Here's how the part is built. I have some questions about the finished solid (model axes, mm). Face numbers are marked on the shaded views. A direction names the side the tool comes from. Give positions to 0.01 mm unless a question says otherwise; leave off trailing zeros. Loops run counter-clockwise (first coordinate to the right, second up) from the corner with the lowest first, then second, coordinate; pieces in that order, holes last.
Q1. Will these pins go through, and if not, where does the flat tip stop? P1, Ø5, axis at y = 4, z = -1, coming from the +X side; P2, Ø1.2, axis at x = 30, y = 22, coming from the +Z side; P3, Ø6.5, axis at y = 20.5, z = -30, coming from the +X side; P4, Ø1.5, axis at x = 50.5, z = -20.5, coming from the -Y side.
Q2. We'd pull the mould along Z, two halves only. Please class the marked faces 1, 2, 3 and 4: +Z half, -Z half, draft (parallel to the pull), parting line (faces both ways), or undercut.
Q3. If we section it at B-B (z = -29.5): Please give me the cut outline in (x, y).
Q4. For the marked faces 5, 6 and 7, which set-ups out of +Z, -Z, +X, -X, +Y, -Y let a thin tool reach every point of the face, with its end or its side?
Q5. I need wall thicknesses on line 1 (Z direction, x = 13.5, y = 8.5); line 2 (Y direction, x = 30, z = 4); line 3 (X direction, y = 20.25, z = -32). Which ranges of each line are inside material? Lowest first, please.
Q6. If we section it at A-A (z = -8): Please give me the cut outline in (x, y).
from build123d import *

# Parameters (mm, degrees)
SALIENTE_EXTRUIR1_DEPTH    = 25
CROQUIS2_W                 = 40
CROQUIS2_H                 = 40
CORTAR_EXTRUIR1_DEPTH      = 20
CORTAR_EXTRUIR2_DEPTH      = 70
CORTAR_EXTRUIR2_DEPTH_BACK = 20
CORTAR_EXTRUIR3_DEPTH      = 42
CORTAR_EXTRUIR3_DEPTH_BACK = 2
CROQUIS8_R                 = 1
CORTAR_EXTRUIR7_DEPTH      = 10
CROQUIS9_R                 = 1
CORTAR_EXTRUIR8_DEPTH      = 10
CROQUIS10_R                = 2
CORTAR_EXTRUIR9_DEPTH      = 1.5
CROQUIS11_R                = 2
CORTAR_EXTRUIR10_DEPTH     = 1.5
CORTAR_EXTRUIR11_DEPTH     = 70
CORTAR_EXTRUIR12_DEPTH     = 10
CORTAR_EXTRUIR13_DEPTH     = 10
CROQUIS14_W                = 3
CROQUIS14_H                = 6
CORTAR_EXTRUIR14_DEPTH     = 14


with BuildPart() as part:
    # Croquis1 → Saliente-Extruir1 (new body)
    with BuildSketch(Plane(origin=(0, 0, 0), x_dir=(1, 0, 0), z_dir=(0, 1, 0))):
        Polygon((-5, 45), (-5, 0), (-5, -5), (125, -5), (125, 45), align=None)
    extrude(amount=SALIENTE_EXTRUIR1_DEPTH)

    # Croquis2 → Cortar-Extruir1 (cut)
    with BuildSketch(Plane(origin=(0, 25, 0), x_dir=(1, 0, 0), z_dir=(0, 1, 0))):
        with Locations((20, 20)):
            Rectangle(CROQUIS2_W, CROQUIS2_H)
    extrude(amount=-CORTAR_EXTRUIR1_DEPTH, mode=Mode.SUBTRACT)

    # Croquis3 → Cortar-Extruir2 (cut, two sides)
    with BuildSketch(Plane.XY.offset(-40)) as cortar_extruir2_sk:
        with BuildLine():
            ThreePointArc((5.5, 15), (10, 19.5), (14.5, 15))
            Line((14.5, 15), (14.5, 25))
            Line((14.5, 25), (5.5, 25))
            Line((5.5, 25), (5.5, 15))
        make_face()
        with BuildLine():
            ThreePointArc((5.5, 15), (10, 10.5), (14.5, 15))
            Line((14.5, 15), (5.5, 15))
        make_face()
        with BuildLine():
            Line((5.5, 15), (14.5, 15))
            ThreePointArc((14.5, 15), (10, 19.5), (5.5, 15))
        make_face()
    extrude(amount=CORTAR_EXTRUIR2_DEPTH, mode=Mode.SUBTRACT)
    extrude(cortar_extruir2_sk.sketch, amount=-CORTAR_EXTRUIR2_DEPTH_BACK, mode=Mode.SUBTRACT)

    # Croquis4 → Cortar-Extruir3 (cut, two sides)
    with BuildSketch(Plane.XY.offset(-40)) as cortar_extruir3_sk:
        with BuildLine():
            Line((14.5, 15), (17, 15))
            ThreePointArc((17, 15), (16.34428877, 17.958039892), (14.5, 20.361902647))
            Line((14.5, 20.361902647), (14.5, 15))
        make_face()
        with BuildLine():
            ThreePointArc((3, 15), (10, 8), (17, 15))
            Line((17, 15), (14.5, 15))
            ThreePointArc((14.5, 15), (10, 10.5), (5.5, 15))
            Line((5.5, 15), (3, 15))
        make_face()
        with BuildLine():
            ThreePointArc((5.5, 20.361902647), (3.65571123, 17.958039892), (3, 15))
            Line((3, 15), (5.5, 15))
            Line((5.5, 15), (5.5, 20.361902647))
        make_face()
        with BuildLine():
            Line((3, 25), (3, 15))
            ThreePointArc((3, 15), (3.65571123, 17.958039892), (5.5, 20.361902647))
            Line((5.5, 20.361902647), (5.5, 25))
            Line((5.5, 25), (3, 25))
        make_face()
        with BuildLine():
            ThreePointArc((14.5, 20.361902647), (16.34428877, 17.958039892), (17, 15))
            Line((17, 15), (17, 25))
            Line((17, 25), (14.5, 25))
            Line((14.5, 25), (14.5, 20.361902647))
        make_face()
    extrude(amount=CORTAR_EXTRUIR3_DEPTH, mode=Mode.SUBTRACT)
    extrude(cortar_extruir3_sk.sketch, amount=-CORTAR_EXTRUIR3_DEPTH_BACK, mode=Mode.SUBTRACT)

    # Croquis8 → Cortar-Extruir7 (cut)
    with BuildSketch(Plane.XY.offset(-40)):
        with Locations((37.5, 22.5)):
            Circle(CROQUIS8_R)
        with Locations((37.5, 7.5)):
            Circle(CROQUIS8_R)
        with Locations((22.5, 7.5)):
            Circle(CROQUIS8_R)
        with Locations((22.5, 22.5)):
            Circle(CROQUIS8_R)
    extrude(amount=-CORTAR_EXTRUIR7_DEPTH, mode=Mode.SUBTRACT)

    # Croquis9 → Cortar-Extruir8 (cut)
    with BuildSketch(Plane(origin=(0, 0, 0), x_dir=(-1, 0, 0), z_dir=(0, 0, -1))):
        with Locations((-30, 22.071067812)):
            Circle(CROQUIS9_R)
        with Locations((-37.071067812, 15)):
            Circle(CROQUIS9_R)
        with Locations((-30, 7.928932188)):
            Circle(CROQUIS9_R)
    extrude(amount=-CORTAR_EXTRUIR8_DEPTH, mode=Mode.SUBTRACT)

    # Croquis10 → Cortar-Extruir9 (cut)
    with BuildSketch(Plane(origin=(0, 0, -45), x_dir=(-1, 0, 0), z_dir=(0, 0, -1))):
        with Locations((-22.5, 22.5)):
            Circle(CROQUIS10_R)
        with Locations((-22.5, 7.5)):
            Circle(CROQUIS10_R)
        with Locations((-37.5, 7.5)):
            Circle(CROQUIS10_R)
        with Locations((-37.5, 22.5)):
            Circle(CROQUIS10_R)
    extrude(amount=-CORTAR_EXTRUIR9_DEPTH, mode=Mode.SUBTRACT)

    # Croquis11 → Cortar-Extruir10 (cut)
    with BuildSketch(Plane.XY.offset(5)):
        with Locations((30, 22.071067812)):
            Circle(CROQUIS11_R)
        with Locations((37.071067812, 15)):
            Circle(CROQUIS11_R)
        with Locations((30, 7.928932188)):
            Circle(CROQUIS11_R)
    extrude(amount=-CORTAR_EXTRUIR10_DEPTH, mode=Mode.SUBTRACT)

    # Croquis6 → Cortar-Extruir11 (cut)
    with BuildSketch(Plane.XY.offset(5)):
        with BuildLine():
            ThreePointArc((45, 14.616328231), (64.430156973, 7.437849736), (85, 5))
            ThreePointArc((85, 5), (105.569843027, 7.437849736), (125, 14.616328231))
            Line((125, 14.616328231), (125, 25))
            Line((125, 25), (45, 25))
            Line((45, 25), (45, 14.616328231))
        make_face()
        with BuildLine():
            ThreePointArc((125, 14.616328231), (105.569843027, 7.437849736), (85, 5))
            Line((85, 5), (115.083217913, 5))
            ThreePointArc((115.083217913, 5), (120.099831147, 6.87798276), (125, 9.041677006))
            Line((125, 9.041677006), (125, 14.616328231))
        make_face()
        with BuildLine():
            ThreePointArc((125, 9.041677006), (120.099831147, 6.87798276), (115.083217913, 5))
            Line((115.083217913, 5), (125, 5))
            Line((125, 5), (125, 9.041677006))
        make_face()
        with BuildLine():
            Line((54.916782087, 5), (85, 5))
            ThreePointArc((85, 5), (64.430156973, 7.437849736), (45, 14.616328231))
            Line((45, 14.616328231), (45, 9.041677006))
            ThreePointArc((45, 9.041677006), (49.900168853, 6.87798276), (54.916782087, 5))
        make_face()
        with BuildLine():
            Line((45, 5), (54.916782087, 5))
            ThreePointArc((54.916782087, 5), (49.900168853, 6.87798276), (45, 9.041677006))
            Line((45, 9.041677006), (45, 5))
        make_face()
    extrude(amount=-CORTAR_EXTRUIR11_DEPTH, mode=Mode.SUBTRACT)

    # Croquis12 → Cortar-Extruir12 (cut)
    with BuildSketch(Plane(origin=(0, 5, 0), x_dir=(1, 0, 0), z_dir=(0, 1, 0))):
        Polygon((108.263538332, 57.3224396), (100, 45), (125, 45), (125, 20), (125, -5), (100, -5), (92.796515759, -13.049468459), (132.437262959, -23.501277263), (155.434902904, 7.824857744), (139.962048677, 54.254841825), align=None)
        with BuildLine():
            Line((125, -5), (125, 20))
            ThreePointArc((125, 20), (117.67766953, 2.32233047), (100, -5))
            Line((100, -5), (125, -5))
        make_face()
        with BuildLine():
            Line((125, 45), (100, 45))
            ThreePointArc((100, 45), (117.67766953, 37.67766953), (125, 20))
            Line((125, 20), (125, 45))
        make_face()
    extrude(amount=-CORTAR_EXTRUIR12_DEPTH, mode=Mode.SUBTRACT)

    # Croquis13 → Cortar-Extruir13 (cut)
    with BuildSketch(Plane(origin=(0, 5, 0), x_dir=(1, 0, 0), z_dir=(0, 1, 0))):
        with BuildLine():
            Line((100, 45), (136.076424828, 53.027802714))
            Line((136.076424828, 53.027802714), (154.686517999, 18.057188076))
            Line((154.686517999, 18.057188076), (135.411120125, -29.058819331))
            Line((135.411120125, -29.058819331), (100, -5))
            add(Edge.make_bspline(
                [(45, -5), (61.631849348, 3.922329445), (83.736441822, 7.63137214), (100, -5)],
                knots=[0, 0, 0, 0, 1, 1, 1, 1], degree=3))
            Line((45, -5), (-2.569566086, -27.480051403))
            Line((-2.569566086, -27.480051403), (140.150106541, -43.115071719))
            Line((140.150106541, -43.115071719), (174.827779806, 24.436234005))
            Line((174.827779806, 24.436234005), (136.076424828, 62.541584801))
            Line((136.076424828, 62.541584801), (45, 45))
            add(Edge.make_bspline(
                [(45, 45), (61.631849348, 36.077670555), (83.736441822, 32.36862786), (100, 45)],
                knots=[0, 0, 0, 0, 1, 1, 1, 1], degree=3))
        make_face()
    extrude(amount=-CORTAR_EXTRUIR13_DEPTH, mode=Mode.SUBTRACT)

    # Croquis14 → Cortar-Extruir14 (cut)
    with BuildSketch(Plane(origin=(0, 25, 0), x_dir=(1, 0, 0), z_dir=(0, 1, 0))):
        with Locations((-1.5, 30)):
            Rectangle(CROQUIS14_W, CROQUIS14_H)
    extrude(amount=-CORTAR_EXTRUIR14_DEPTH, mode=Mode.SUBTRACT)


solid = part.part
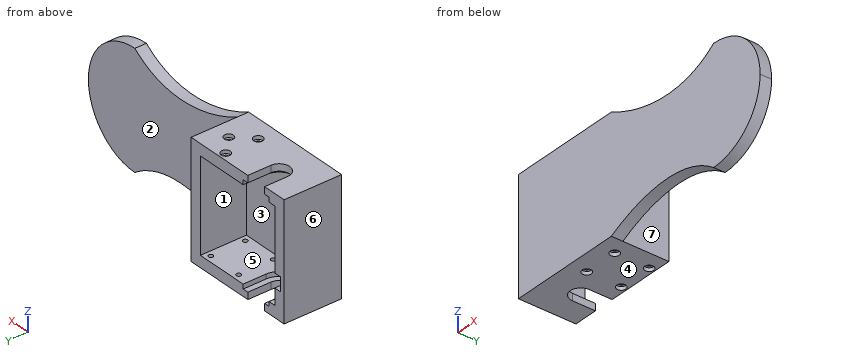
Check sheet entries:
1. P1: stops at x = 118.78
1. P2: stops at z = -40
1. P3: stops at x = 45
1. P4: stops at y = 0
2. face 1: undercut
2. face 2: draft
2. face 3: undercut
2. face 4: -Z half
3. outline: (-5, 0) - (123.12, 0) - (123.12, 5) - (45, 5) - (45, 25) - (40, 25) - (40, 5) - (0, 5) - (0, 11) - (-3, 11) - (-3, 25) - (-5, 25) - close
4. face 5: +Y
4. face 6: +Z, -Z, -X, +Y, -Y
4. face 7: +Z, -Z, +X, +Y
5. line 1: z = -45 to -40, 0 to 5
5. line 2: y = 0 to 5.93, 9.93 to 20.07, 24.07 to 25
5. line 3: x = -5 to -3, 40 to 45
6. outline: (-5, 0) - (121.93, 0) - (121.93, 5) - (45, 5) - (45, 25) - (40, 25) - (40, 5) - (0, 5) - (0, 25) - (-5, 25) - close
